from build123d import *

# Parameters (mm, degrees)
SKETCH1_R           = 1.25
BOSS_EXTRUDE1_DEPTH = 1.25
SCALE1_SCALE        = 1.5


with BuildPart() as part:
    # Sketch1 → Boss-Extrude1 (new body)
    with BuildSketch(Plane.XY):
        Polygon((1.868889761, -1.070364136), (1.861407413, 1.083323942), (-0.007482348, 2.153688078), (-1.868889761, 1.070364136), (-1.861407413, -1.083323942), (0.007482348, -2.153688078), align=None)
        Circle(SKETCH1_R, mode=Mode.SUBTRACT)
    extrude(amount=BOSS_EXTRUDE1_DEPTH)


with BuildPart() as part_1:
    # Scale1: scaled about (0, 0, 0.625)
    add(part.part.scale(SCALE1_SCALE).moved(Location((0, 0, -0.3125))))


solid = part_1.part
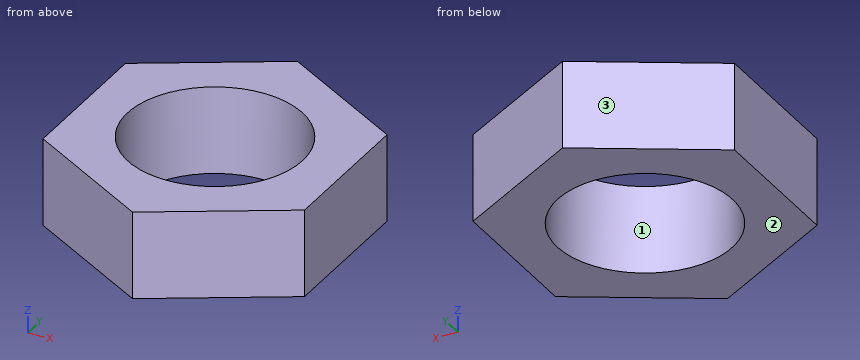
Read the model definition and answer for the solid it produces. Units are mm, in the model's axes. Face numbers are marked on the shaded views. Round coordinates to 2 decimals unless told otherwise and drop trailing zeros. Loops run counter-clockwise (first coordinate to the right, second up) from the corner with the lowest first, then second, coordinate; pieces in that order, holes last.
Q1. Section C-C on y = -0.5 is taken. Write down the section's boundary in (x, z).
Q2. Section A-A on z = 0.65 is taken. Write down the section's boundary in (x, y) (3 decimals), and give its area (3 significant figures).
Q3. Consider probe 1 along Y at (x, z) = (-1.6, 0.8); probe 2 along X at (y, z) = (-1, 0.2); probe 3 along X at (y, z) = (-0.75, 0). Determine where each line is inside the solid, lowest interval first.
Q4. Determine the mould class of the marked faces 1, 2 and 3 for opening direction X: released by +X, released by -X, zero draft, split by the parting line, or undercut.
Q5. Section B-B on x = 0.2 is taken. Write down the section's boundary in (y, z).
Q6. This flat-tipped pin is pushed along its axis until it touches: pin 1 (3 mm diameter, centred on x = -0.5, y = 0, fed in from -Z). Where does it stop, or does it pass through?
Output:
1. outline: (-2.8, -0.31) - (-1.81, -0.31) - (-1.81, 1.56) - (-2.8, 1.56) - close; (1.81, -0.31) - (2.8, -0.31) - (2.8, 1.56) - (1.81, 1.56) - close
2. outline: (-2.803, 1.606) - (-2.792, -1.625) - (0.011, -3.231) - (2.803, -1.606) - (2.792, 1.625) - (-0.011, 3.231) - close; hole circle Ø3.75 at (0, 0)
2. area: 16.1 mm2
3. probe 1: y = -2.31 to -0.98, 0.98 to 2.31
3. probe 2: x = -2.79 to -1.59, 1.59 to 2.8
3. probe 3: x = -2.8 to -1.72, 1.72 to 2.8
4. face 1: undercut
4. face 2: zero draft
4. face 3: released by -X
5. outline: (-3.12, -0.31) - (-1.86, -0.31) - (-1.86, 1.56) - (-3.12, 1.56) - close; (1.86, -0.31) - (3.11, -0.31) - (3.11, 1.56) - (1.86, 1.56) - close
6. pin 1: stops at z = -0.31
